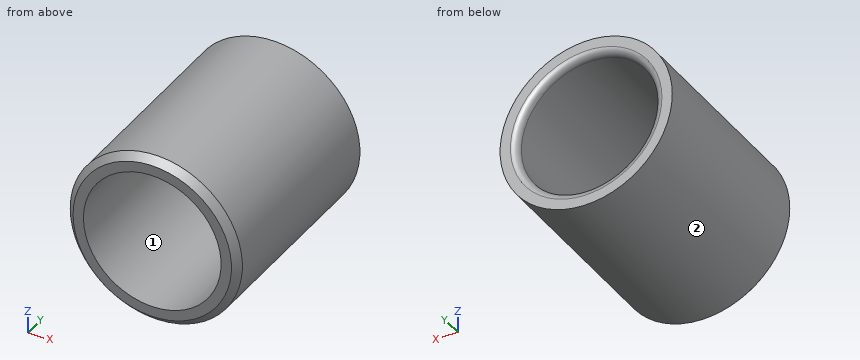
from build123d import *

# Parameters (mm, degrees)
BODY_SECTION_W      = 1.5875
BODY_SECTION_H      = 19.05
TOP_RADIUS_R        = 0.635
BOTTOM_CHAMFER_SIZE = 0.635


with BuildPart() as part:
    # BODY SECTION → BODY (revolve)
    with BuildSketch(Plane.XY, mode=Mode.PRIVATE) as body_sk:
        with Locations((7.14375, -9.525)):
            Rectangle(BODY_SECTION_W, BODY_SECTION_H)
    revolve(body_sk.sketch.rotate(Axis((0, 0, 0), (0, -1, 0)), 180), axis=Axis((0, 0, 0), (0, -1, 0)))

    # TOP RADIUS
    top_radius_edges = [part.edges().sort_by_distance(p)[0] for p in [
        (6.35, 0, 0),
    ]]
    fillet(top_radius_edges, radius=TOP_RADIUS_R)

    # BOTTOM CHAMFER
    bottom_chamfer_edges = [part.edges().sort_by_distance(p)[0] for p in [
        (7.9375, -19.05, 0),
    ]]
    chamfer(bottom_chamfer_edges, length=BOTTOM_CHAMFER_SIZE)


solid = part.part
Geometry: final body of the model. Coordinates: model frame, mm. Face numbers are marked on the shaded views. Coordinates: 2 decimals unless noted, no trailing zeros.
(1) Material intervals for probe 1 along Z at (x, y) = (0, -7.75); probe 2 along Z at (x, y) = (1.5, -8.25); probe 3 along X at (y, z) = (-1, 5.5), sorted ascending.
(2) First-contact query: pin 1 (1.5 mm diameter, centred on x = -2.5, y = -15, fed in from -Z); pin 2 (1 mm diameter, centred on y = -17, z = 1, fed in from +X); pin 3 (2 mm diameter, centred on y = -4, z = 2.5, fed in from -X). Flat tips, straight axial feed; report the tip coordinate or a pass-through.
(3) Draft query along X for the marked faces 1 and 2. Return one class per face: pulls with the +X half, pulls with the -X half, needs draft (parallel to the pull), parting line crosses it, or undercut.
Solution:
1. probe 1: z = -7.94 to -6.35, 6.35 to 7.94
1. probe 2: z = -7.79 to -6.17, 6.17 to 7.79
1. probe 3: x = -5.72 to -3.17, 3.17 to 5.72
2. pin 1: stops at z = -7.74
2. pin 2: stops at x = 7.92
2. pin 3: stops at x = -7.79
3. face 1: undercut
3. face 2: parting line crosses it
